Source: three-view drawing plus pictorial views. Frame: mm from the lowest corner of the part. A direction names the side the tool comes from. Round coordinates to 2 decimals unless told otherwise and drop trailing zeros. Order: outer loops, then holes, each group sorted by start corner. A loop starts at its lowest first (then second) coordinate and runs counter-clockwise, first axis right, second up. Notation, with made-up numbers: (33.25, -28.75) -> (55.25, -28.75) arc R4 cw to (55.25, -21.75) -> close; hole circle Ø9 at (25, 89). An arc over 180 degrees is marked (long way). Answer as CSV lines item,"result".
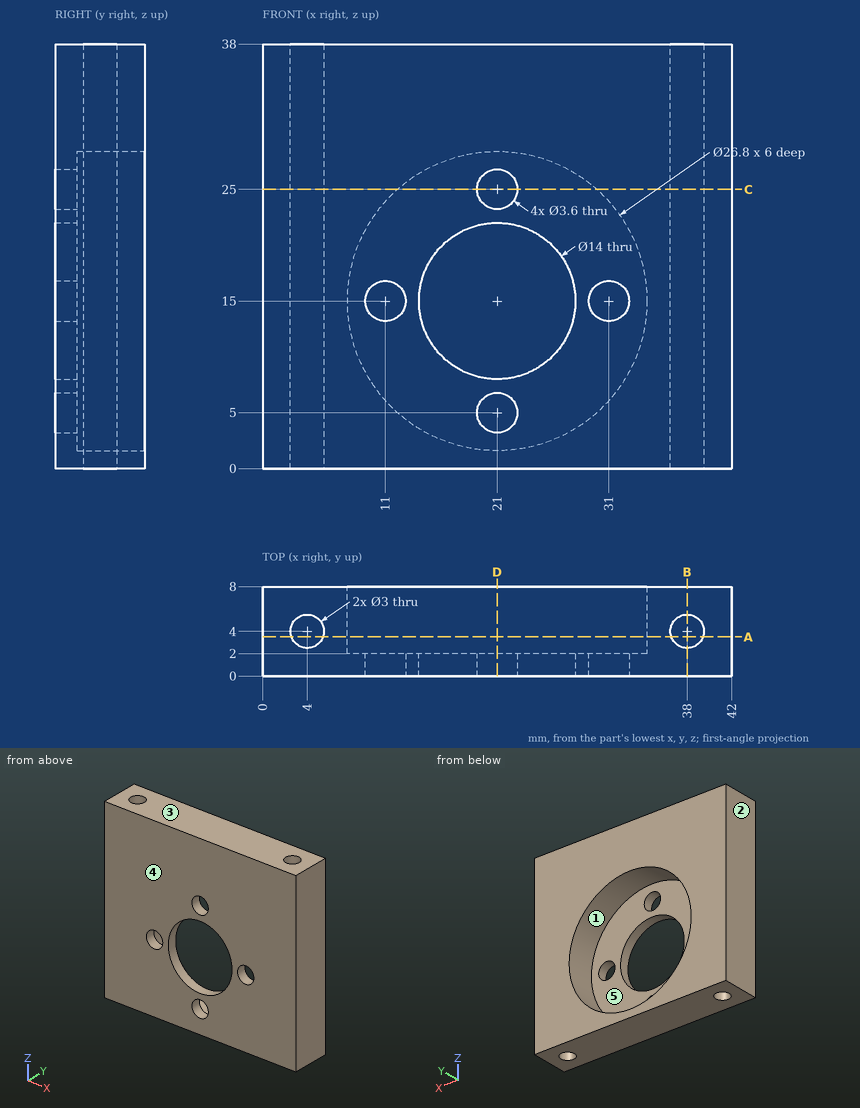
1. Section query D-D on x = 21. Return loops of the section in (y, z).
Results below:
outline,"(0, 0) -> (8, 0) -> (8, 1.6) -> (2, 1.6) -> (2, 3.2) -> (0, 3.2) -> close; (0, 6.8) -> (2, 6.8) -> (2, 8) -> (0, 8) -> close; (0, 22) -> (2, 22) -> (2, 23.2) -> (0, 23.2) -> close; (0, 26.8) -> (2, 26.8) -> (2, 28.4) -> (8, 28.4) -> (8, 38) -> (0, 38) -> close"
2. Section query A-A on y = 3.5. Return loops of the section in (x, z), and give its area (3 significant figures).
Results below:
outline,"(0, 0) -> (2.59, 0) -> (2.59, 38) -> (0, 38) -> close; (5.41, 0) -> (36.59, 0) -> (36.59, 38) -> (5.41, 38) -> close; (39.41, 0) -> (42, 0) -> (42, 38) -> (39.41, 38) -> close; hole circle Ø26.8 at (21, 15)"
area,"817 mm2"
3. Reachability of the marked faces 1 and 2 from +Z, -Z, +X, -X, +Y, -Y: full face, straight path, thin tool, end or side. Return the list, or none.
Results below:
face 1,"+Y"
face 2,"+Z, -Z, -X, +Y, -Y"
4. Line query: L1, parallel to Z at x = 21, y = 0.9; L2, parallel to Z at x = 31, y = 1.25; L3, parallel to X at y = 2.75, z = 30. Output: solid intervals per line, ascending. Write a range as [from, to].
Results below:
L1,"[0, 3.2], [6.8, 8], [22, 23.2], [26.8, 38]"
L2,"[0, 13.2], [16.8, 38]"
L3,"[0, 3.17], [4.83, 37.17], [38.83, 42]"
5. Section query B-B on x = 38. Return loops of the section in (y, z), and give its area (3 significant figures).
Results below:
outline,"(0, 0) -> (2.5, 0) -> (2.5, 38) -> (0, 38) -> close; (5.5, 0) -> (8, 0) -> (8, 38) -> (5.5, 38) -> close"
area,"190 mm2"
6. Mould query, pull axis Z, two halves, no side actions, for the marked faces 3, 4 and 5. Classes: released by +Z, released by -Z, zero draft, split by the parting line, or undercut.
Results below:
face 3,"released by +Z"
face 4,"zero draft"
face 5,"undercut"
7. Section query C-C on z = 25. Return loops of the section in (x, y).
Results below:
outline,"(0, 0) -> (19.2, 0) -> (19.2, 2) -> (12.08, 2) -> (12.08, 8) -> (0, 8) -> close; (22.8, 0) -> (42, 0) -> (42, 8) -> (29.92, 8) -> (29.92, 2) -> (22.8, 2) -> close; hole circle Ø3 at (4, 4); hole circle Ø3 at (38, 4)"
8. Pin query (flat end, axial travel): pin 1 (1 mm diameter, centred on x = 30, z = 5.5, fed in from -Y); pin 2 (18 mm diameter, centred on x = 21, z = 15, fed in from +Y). Return the tip coordinate at first contact, or that it passes through.
Results below:
pin 1,"y = 0"
pin 2,"y = 2"
